Model file for the job. Use its own axes, mm. Face numbers are marked on the shaded views. A direction names the side the tool comes from. Coordinates: 2 decimals unless noted, no trailing zeros. Write each loop counter-clockwise with the first axis right and the second up, starting at its lowest first coordinate (ties: lowest second). Pieces come first, ordered by that corner, then holes. Notation, with made-up numbers: (60, 82.25) - (84, 82.25) arc R18 ccw to (84, 104.25) - close; hole circle Ø1 at (-17, 24). An arc over 180 degrees is marked (long way). Put each result on its own line as item: value. Start each with the question number.
1. Which spindle directions (+Z, -Z, +X, -X, +Y, -Y) get a long thin tool onto all of the face, cutting with end or side? Do the marked faces 1 and 2. Say none if no direction does.
2. Drill centre lines: L1, parallel to X at y = 4.1, z = 0; L2, parallel to X at y = 2.1, z = 0; L3, parallel to Z at x = 2.5, y = 0.45. Where is each one in solid material? Low to high. Write a range as from..to.
3. Saw through at C-C, the plane y = 2.1. Write the cut outline in (x, z).
4. Pull direction Z, two halves, no side cores. Call the marked faces 3, 4 and 5: released by +Z, released by -Z, zero draft, split by the parting line, or undercut.
5. Drop a flat-ended pin along its axis: P1, Ø2, axis at x = 4, y = 2.5, coming from the -Z side. Give the stop position or say it passes through.
```python
from build123d import *

# Parameters (mm, degrees)
SKETCH_1_R      = 5
SKETCH_1_R_2    = 3.65
EXTRUDE_1_DEPTH = 3.3
SKETCH_2_R      = 5.5
SKETCH_2_R_2    = 3.55
EXTRUDE_2_DEPTH = 1
EXTRUDE_START   = 1
SKETCH_3_R      = 5.5
SKETCH_3_R_2    = 3.55
EXTRUDE_3_DEPTH = 1
CHAMFER_1_SIZE  = 0.5


with BuildPart() as part:
    # 草图1 → 凸台-拉伸1 (new body)
    with BuildSketch(Plane(origin=(0, 0, 0), x_dir=(1, 0, 0), z_dir=(0, 1, 0))):
        with Locations(Location((0, 0, 0), (0, 0, 270))):
            Circle(SKETCH_1_R)
        with Locations(Location((0, 0, 0), (0, 0, 270))):
            Circle(SKETCH_1_R_2, mode=Mode.SUBTRACT)
    extrude(amount=EXTRUDE_1_DEPTH)

    # 草图2 → 凸台-拉伸2 (add)
    with BuildSketch(Plane.XZ):
        with Locations(Location((0, 0, 0), (0, 0, 270))):
            Circle(SKETCH_2_R)
        with Locations(Location((0, 0, 0), (0, 0, 270))):
            Circle(SKETCH_2_R_2, mode=Mode.SUBTRACT)
    extrude(amount=EXTRUDE_2_DEPTH)

    # 草图3 → 凸台-拉伸3 (add)
    with BuildSketch(Plane(origin=(0, 3.3, 0), x_dir=(1, 0, 0), z_dir=(0, 1, 0)).offset(EXTRUDE_START)):
        with Locations(Location((0, 0, 0), (0, 0, 90))):
            Circle(SKETCH_3_R)
        with Locations(Location((0, 0, 0), (0, 0, 90))):
            Circle(SKETCH_3_R_2, mode=Mode.SUBTRACT)
    extrude(amount=-EXTRUDE_3_DEPTH)

    # 倒角1
    chamfer_1_edges = [part.edges().sort_by_distance(p)[0] for p in [
        (0, 0, 5.5),
        (0, 3.3, 5.5),
    ]]
    chamfer(chamfer_1_edges, length=CHAMFER_1_SIZE - 0.0001)  # a hair under: the kernel refuses the full size


solid = part.part
```
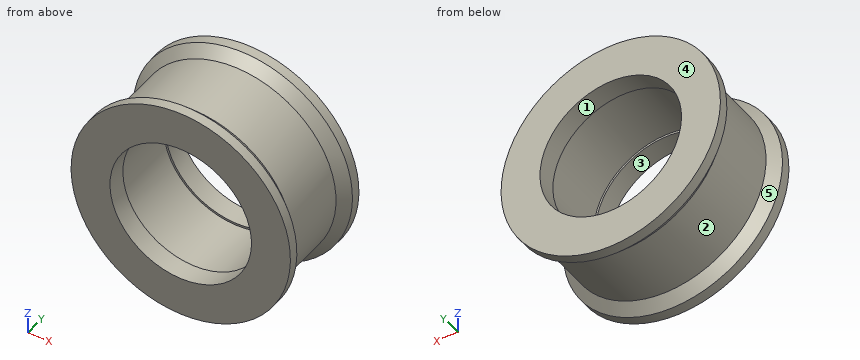
Final values:
1. face 1: +Y, -Y
1. face 2: none
2. L1: x = -5.5..-3.55, 3.55..5.5
2. L2: x = -5..-3.65, 3.65..5
2. L3: z = -4.33..-2.66, 2.66..4.33
3. outline: circle Ø10 at (0, 0); hole circle Ø7.3 at (0, 0)
4. face 3: undercut
4. face 4: zero draft
4. face 5: split by the parting line
5. P1: stops at z = -4
